```python
from build123d import *


with BuildPart() as part:
    # SK_Wheel → Wheel (revolve)
    with BuildSketch(Plane(origin=(0, 0, 0), x_dir=(1, 0, 0), z_dir=(0, 1, 0)), mode=Mode.PRIVATE) as wheel_sk:
        Polygon((0, 13), (12, 13), (12, 8), (38, 8), (38, 13), (50, 13), (50, -13), (38, -13), (38, -8), (12, -8), (12, -13), (0, -13), align=None)
    revolve(wheel_sk.sketch.rotate(Axis((0, 0, -18), (0, 0, 1)), 180), axis=Axis((0, 0, -18), (0, 0, 1)))


solid = part.part
```
Read the model definition and answer for the solid it produces. Units are mm, in the model's axes. A direction names the side the tool comes from. Give positions to 0.01 mm unless a question says otherwise; leave off trailing zeros. Write each loop counter-clockwise with the first axis right and the second up, starting at its lowest first coordinate (ties: lowest second). Pieces come first, ordered by that corner, then holes. Notation, with made-up numbers: (28.5, -29) -> (36.5, -29) arc R18 cw to (36.5, -25) -> close; hole circle Ø3 at (-18.5, 42). An arc over 180 degrees is marked (long way). Answer in a Markdown table with one row per item.
1) Section D-D on z = -4.5 is taken. Give the vertices of the cut face in (x, y).
Results list:
| item | result |
|---|---|
| outline | circle Ø100 at (0, 0) |
2) Straight lines are drawn through the part: line 1 (Y direction, x = 0, z = 10.8); line 2 (Y direction, x = 7.5, z = -8.75); line 3 (Z direction, x = -26, y = -10.5). For each, find the intervals that lie inside material, in ascending order. Write a range as [from, to].
Results list:
| item | result |
|---|---|
| line 1 | [-50, -38], [-12, 12], [38, 50] |
| line 2 | [-49.43, -37.25], [-9.37, 9.37], [37.25, 49.43] |
| line 3 | [-8, 8] |
3) Section A-A on x = 0 is taken. Give the vertices of the cut face in (y, z).
Results list:
| item | result |
|---|---|
| outline | (-50, -13) -> (-38, -13) -> (-38, -8) -> (-12, -8) -> (-12, -13) -> (12, -13) -> (12, -8) -> (38, -8) -> (38, -13) -> (50, -13) -> (50, 13) -> (38, 13) -> (38, 8) -> (12, 8) -> (12, 13) -> (-12, 13) -> (-12, 8) -> (-38, 8) -> (-38, 13) -> (-50, 13) -> close |
4) Section C-C on y = 8 is taken. Give the vertices of the cut face in (x, z).
Results list:
| item | result |
|---|---|
| outline | (-49.36, -13) -> (-37.15, -13) -> (-37.15, -8) -> (-8.94, -8) -> (-8.94, -13) -> (8.94, -13) -> (8.94, -8) -> (37.15, -8) -> (37.15, -13) -> (49.36, -13) -> (49.36, 13) -> (37.15, 13) -> (37.15, 8) -> (8.94, 8) -> (8.94, 13) -> (-8.94, 13) -> (-8.94, 8) -> (-37.15, 8) -> (-37.15, 13) -> (-49.36, 13) -> close |
5) A tool of negligible diameter and unlimited length cuts with its end or side. For faces 4 (the cylindrical face through (8.238, 37.096, 10.465)), 5 (the flat face through (-11, -37, 13)), 6 (the flat face through (-9, -9, -8)), from which of +Z, -Z, +X, -X, +Y, -Y can it reach the whole face along a straight path? Write none if from no direction.
Results list:
| item | result |
|---|---|
| face 4 | +Z |
| face 5 | +Z, +X, -X, +Y, -Y |
| face 6 | -Z |
6) Each of these flat-tipped pins is pushed along its axis until it touches: pin 1 Ø5 at (x, z) = (35, -4.5) entering from -Y; pin 2 Ø5 at (x, z) = (-26, 10) entering from +Y; pin 3 Ø12 at (y, z) = (7, -7.5) entering from +X. Where does it stop, or does it pass through?
Results list:
| item | result |
|---|---|
| pin 1 | y = -38 |
| pin 2 | y = 44.13 |
| pin 3 | x = 49.99 |
7) Determine the mould class of faces 1 (the flat face through (0, 0, 13)), 2 (the cylindrical face through (-47.69, -15.02, 0.18)), 3 (the cylindrical face through (-11.446, -3.604, 10.535)) for opening direction Y: released by +Y, released by -Y, zero draft, split by the parting line, or undercut.
Results list:
| item | result |
|---|---|
| face 1 | zero draft |
| face 2 | split by the parting line |
| face 3 | undercut |
8) Section B-B on z = 10.5 is taken. Give the vertices of the cut face in (x, y), plus the area to 3 significant figures.
Results list:
| item | result |
|---|---|
| outline | circle Ø100 at (0, 0); circle Ø24 at (0, 0); hole circle Ø76 at (0, 0) |
| area | 3,770 mm^2 |
